Here's how the part is built. I have some questions about the finished solid (model axes, mm). Coordinates: 2 decimals unless noted, no trailing zeros. Loops run counter-clockwise (first coordinate to the right, second up) from the corner with the lowest first, then second, coordinate; pieces in that order, holes last. Notation, with made-up numbers: M 84.25,82 L 142.25,82 A23 ccw 142.25,121 Z; hole C 32.5,72 d2. An arc over 180 degrees is marked long. Use one line per item in the form item = value. Start each with the question number.
(1) Imagine slicing it at A-A, the plane y = 4. Please give me the cut outline in (x, z) (3 decimals), and give its area (3 significant figures).
(2) Imagine slicing it at B-B, the plane x = -69.85. Please give me the cut outline in (y, z), and give its area (3 significant figures).
(3) Please list where these lines run through material, in increasing order: L1, parallel to X at y = 1.5, z = -12.7; L2, parallel to X at y = 2, z = 0; L3, parallel to Z at x = -55.5, y = 5.25.
(4) Imagine slicing it at D-D, the plane z = -2.5. Please give me the cut outline in (x, y), and give its area (3 significant figures).
(5) Will this pin go through, and if not, where does the flat tip stop? P1, Ø1.5, axis at y = 1.5, z = -8.5, coming from the +X side.
(6) Imagine slicing it at C-C, the plane x = 6.35. Please give me the cut outline in (y, z) (3 decimals), and give its area (3 significant figures).
```python
from build123d import *

# Parameters (mm, degrees)
SKETCH1_W           = 152.4
SKETCH1_H           = 88.9
SKETCH1_R           = 3.429
BOSS_EXTRUDE1_DEPTH = 6.35
CUT_EXTRUDE3_START  = 6.35
SKETCH2_R           = 16.25
SKETCH2_R_2         = 13.5
CUT_EXTRUDE3_DEPTH  = 4.25
SKETCH3_W           = 76.2
SKETCH3_H           = 19.05
CUT_EXTRUDE4_DEPTH  = 89.44526556
SKETCH4_OUTSIDE_W   = 189.71
SKETCH4_OUTSIDE_H   = 126.21
SKETCH4_OUTSIDE_W_2 = 101.6
SKETCH4_OUTSIDE_H_2 = 50.8
CUT_EXTRUDE6_DEPTH  = 89.44526556


with BuildPart() as part:
    # Sketch1 → Boss-Extrude1 (new body)
    with BuildSketch(Plane(origin=(0, 0, 0), x_dir=(1, 0, 0), z_dir=(0, 1, 0))):
        Rectangle(SKETCH1_W, SKETCH1_H)
        with Locations(Location((-69.85, 38.1, 0), (0, 0, 270))):
            Circle(SKETCH1_R, mode=Mode.SUBTRACT)
        with Locations(Location((-57.15, 38.1, 0), (0, 0, 270))):
            Circle(SKETCH1_R, mode=Mode.SUBTRACT)
        with Locations(Location((-57.15, 25.4, 0), (0, 0, 270))):
            Circle(SKETCH1_R, mode=Mode.SUBTRACT)
        with Locations(Location((-57.15, 12.7, 0), (0, 0, 270))):
            Circle(SKETCH1_R, mode=Mode.SUBTRACT)
        with Locations(Location((-57.15, 0, 0), (0, 0, 270))):
            Circle(SKETCH1_R, mode=Mode.SUBTRACT)
        with Locations(Location((-57.15, -12.7, 0), (0, 0, 270))):
            Circle(SKETCH1_R, mode=Mode.SUBTRACT)
        with Locations(Location((-57.15, -25.4, 0), (0, 0, 270))):
            Circle(SKETCH1_R, mode=Mode.SUBTRACT)
        with Locations(Location((-57.15, -38.1, 0), (0, 0, 270))):
            Circle(SKETCH1_R, mode=Mode.SUBTRACT)
        with Locations(Location((-69.85, 25.4, 0), (0, 0, 270))):
            Circle(SKETCH1_R, mode=Mode.SUBTRACT)
        with Locations(Location((-69.85, 12.7, 0), (0, 0, 270))):
            Circle(SKETCH1_R, mode=Mode.SUBTRACT)
        with Locations(Location((-69.85, 0, 0), (0, 0, 270))):
            Circle(SKETCH1_R, mode=Mode.SUBTRACT)
        with Locations(Location((-69.85, -12.7, 0), (0, 0, 270))):
            Circle(SKETCH1_R, mode=Mode.SUBTRACT)
        with Locations(Location((-69.85, -25.4, 0), (0, 0, 270))):
            Circle(SKETCH1_R, mode=Mode.SUBTRACT)
        with Locations(Location((-69.85, -38.1, 0), (0, 0, 270))):
            Circle(SKETCH1_R, mode=Mode.SUBTRACT)
    extrude(amount=BOSS_EXTRUDE1_DEPTH)

    # Sketch2 → Cut-Extrude3 (cut)
    with BuildSketch(Plane(origin=(0, 0, 0), x_dir=(1, 0, 0), z_dir=(0, 1, 0)).offset(CUT_EXTRUDE3_START)):
        with Locations(Location((6.35, 0, 0), (0, 0, 90))):
            Circle(SKETCH2_R)
        with Locations(Location((6.35, 0, 0), (0, 0, 90))):
            Circle(SKETCH2_R_2, mode=Mode.SUBTRACT)
    extrude(amount=-CUT_EXTRUDE3_DEPTH, mode=Mode.SUBTRACT)

    # Sketch3 → Cut-Extrude4 (cut, through all)
    with BuildSketch(Plane(origin=(0, 6.35, 0), x_dir=(1, 0, 0), z_dir=(0, 1, 0))):
        with Locations((38.1, 0)):
            Rectangle(SKETCH3_W, SKETCH3_H)
    extrude(amount=-CUT_EXTRUDE4_DEPTH, mode=Mode.SUBTRACT)

    # Sketch4 outside → Cut-Extrude6 (cut, through all)
    with BuildSketch(Plane(origin=(0, 0, 0), x_dir=(1, 0, 0), z_dir=(0, 1, 0))):
        Rectangle(SKETCH4_OUTSIDE_W, SKETCH4_OUTSIDE_H)
        with Locations((-25.4, 0)):
            Rectangle(SKETCH4_OUTSIDE_W_2, SKETCH4_OUTSIDE_H_2, mode=Mode.SUBTRACT)
    extrude(amount=CUT_EXTRUDE6_DEPTH, mode=Mode.SUBTRACT)


solid = part.part
```
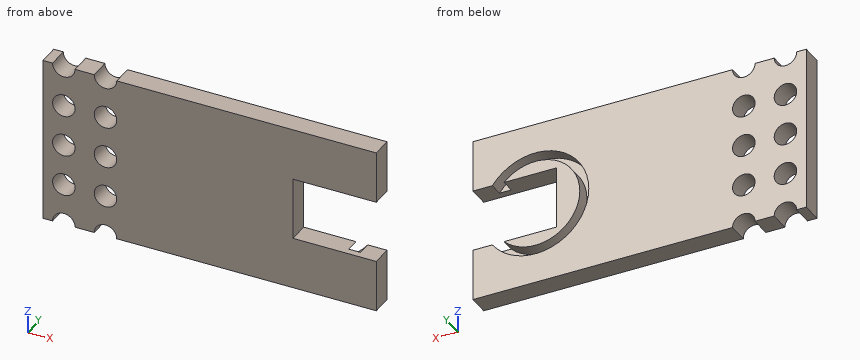
Answer:
q1.outline = M -76.2,-25.4 L -73.279,-25.4 A3.429 cw -66.421,-25.4 L -60.579,-25.4 A3.429 cw -53.721,-25.4 L 25.4,-25.4 L 25.4,-9.525 L 19.516,-9.525 A16.25 cw long 19.516,9.525 L 25.4,9.525 L 25.4,25.4 L -53.721,25.4 A3.429 cw -60.579,25.4 L -66.421,25.4 A3.429 cw -73.279,25.4 L -76.2,25.4 Z; M 0,-9.525 L 0,9.525 L 15.917,9.525 A13.5 ccw long 15.917,-9.525 Z; hole C -69.85,-12.7 d6.858; hole C -69.85,0 d6.858; hole C -69.85,12.7 d6.858; hole C -57.15,-12.7 d6.858; hole C -57.15,0 d6.858; hole C -57.15,12.7 d6.858
q1.area = 4,180 mm²
q2.outline = M 0,-21.97 L 6.35,-21.97 L 6.35,-16.13 L 0,-16.13 Z; M 0,-9.27 L 6.35,-9.27 L 6.35,-3.43 L 0,-3.43 Z; M 0,3.43 L 6.35,3.43 L 6.35,9.27 L 0,9.27 Z; M 0,16.13 L 6.35,16.13 L 6.35,21.97 L 0,21.97 Z
q2.area = 148 mm²
q3.L1 = -76.2 to -73.28, -66.42 to -60.58, -53.72 to 25.4
q3.L2 = -76.2 to -73.28, -66.42 to -60.58, -53.72 to 0
q3.L3 = -22.39 to -15.71, -9.69 to -3.01, 3.01 to 9.69, 15.71 to 22.39
q4.outline = M -76.2,0 L -72.2,0 L -72.2,6.35 L -76.2,6.35 Z; M -67.5,0 L -59.5,0 L -59.5,6.35 L -67.5,6.35 Z; M -54.8,0 L 0,0 L 0,6.35 L -6.92,6.35 L -6.92,2.1 L -9.71,2.1 L -9.71,6.35 L -54.8,6.35 Z
q4.area = 412 mm²
q5.P1 = 0
q6.outline = M 0,-25.4 L 6.35,-25.4 L 6.35,-16.25 L 2.1,-16.25 L 2.1,-13.5 L 6.35,-13.5 L 6.35,-9.525 L 0,-9.525 Z; M 0,9.525 L 6.35,9.525 L 6.35,13.5 L 2.1,13.5 L 2.1,16.25 L 6.35,16.25 L 6.35,25.4 L 0,25.4 Z
q6.area = 178 mm²
